Geometry: see drawing. Coordinates: mm, zero at the bounding-box minimum. A direction names the side the tool comes from. Round coordinates to 2 decimals unless told otherwise and drop trailing zeros. Loops run counter-clockwise (first coordinate to the right, second up) from the corner with the lowest first, then second, coordinate; pieces in that order, holes last. Notation, with made-up numbers: M 42.25,20 L 95.25,20 A11 cw 95.25,39 Z; hole C 73,-16.75 d10. An arc over 180 degrees is marked long. Answer as a JSON object with one key per item and string values.
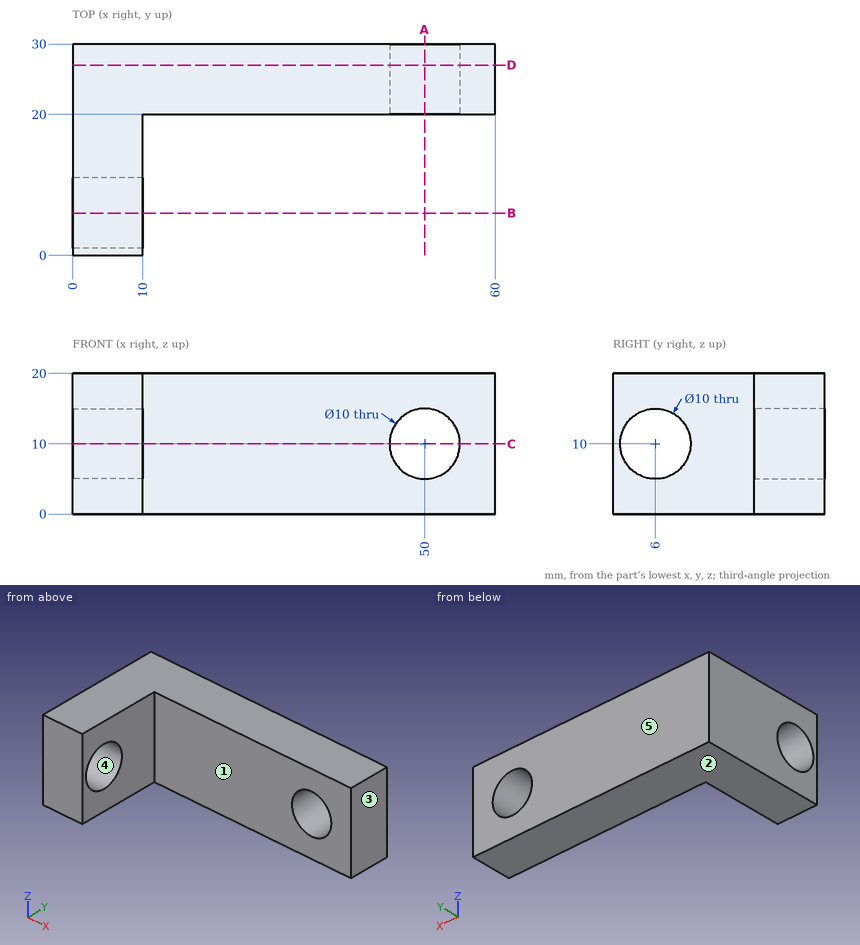
1) Section query B-B (y = 6). Return the cut outline in (x, z), and give its area (3 significant figures).
Results:
{"outline": "M 0,0 L 10,0 L 10,5 L 0,5 Z; M 0,15 L 10,15 L 10,20 L 0,20 Z", "area": "100 mm2"}
2) Ray query, line 1 (X direction, y = 25.75, z = 10); line 2 (Y direction, x = 8.5, z = 10); line 3 (Y direction, x = 29, z = 18.5). Return the intervals inside material, ascending.
Results:
{"line 1": "0 to 45, 55 to 60", "line 2": "0 to 1, 11 to 30", "line 3": "20 to 30"}
3) Reachability of the marked faces 1 and 2 from +Z, -Z, +X, -X, +Y, -Y: full face, straight path, thin tool, end or side. Return the list, or none.
Results:
{"face 1": "+Z, -Z, +X, -Y", "face 2": "-Z, +X, -X, +Y, -Y"}
4) Pull-direction query (Y, two-part tool) for the marked faces 3, 4 and 5; classes: +Y half, -Y half, draft (parallel to the pull), parting line (faces both ways), or undercut.
Results:
{"face 3": "draft", "face 4": "undercut", "face 5": "+Y half"}
5) Section query D-D (y = 27). Return the cut outline in (x, z), and give its area (3 significant figures).
Results:
{"outline": "M 0,0 L 60,0 L 60,20 L 0,20 Z; hole C 50,10 d10", "area": "1,120 mm2"}
6) Section query A-A (x = 50). Return the cut outline in (y, z), and give its area (3 significant figures).
Results:
{"outline": "M 20,0 L 30,0 L 30,5 L 20,5 Z; M 20,15 L 30,15 L 30,20 L 20,20 Z", "area": "100 mm2"}
7) Pin query (flat end, axial travel): P1, Ø8, axis at y = 4, z = 17, coming from the +X side; P2, Ø1.5, axis at x = 26.5, z = 15.5, coming from the -Y side. Return the tip coordinate at first contact, or that it passes through.
Results:
{"P1": "x = 10", "P2": "y = 20"}
8) Section query C-C (z = 10). Return the cut outline in (x, y), and give its area (3 significant figures).
Results:
{"outline": "M 0,0 L 10,0 L 10,1 L 0,1 Z; M 0,11 L 10,11 L 10,20 L 45,20 L 45,30 L 0,30 Z; M 55,20 L 60,20 L 60,30 L 55,30 Z", "area": "600 mm2"}
